The model under review builds one solid part; all positions refer to its coordinate system, in mm. Coordinates: 2 decimals unless noted, no trailing zeros. Write each loop counter-clockwise with the first axis right and the second up, starting at its lowest first coordinate (ties: lowest second). Pieces come first, ordered by that corner, then holes. Notation, with made-up numbers: (50, -3) - (67, -3) arc R33 ccw to (67, 36) - close; hole circle Ø3 at (49.5, 25.25). An arc over 180 degrees is marked (long way). Return JSON: item names as keys, results as strings. Group by question number.
(1) To check wall thickness, follow L1, parallel to X at y = -130, z = 2.35; L2, parallel to Y at x = -28.25, z = 1.2; L3, parallel to Y at x = -85.25, z = 0.8. State the ranges of each line that lie inside material, in increasing order. Write a range as from..to.
(2) We need section A-A on x = 55.5. State the section outline as (y, z) points.
(3) We need section C-C on x = -6. State the section outline as (y, z) points, then the cut area to 3 significant figures.
(4) For pin 1 Ø2.5 at (x, y) = (-85.25, -130) entering from +Z; pin 2 Ø5 at (x, y) = (85.25, 0) entering from +Z, all flat-tipped, find the tip position at first contact; note any pin that passes through.
(5) We need section B-B on z = 0.6. Give the number of separate pieces and of enclosed holes in the cut face, then the cut area to 3 significant figures.
(6) Draft analysis for pull direction Y (two halves, no side actions). For faces 1 (the face through (-1, 2, 3)), 2 (the face through (-1.951, -81.214, 1.479)), state which applies: released by +Y, released by -Y, zero draft, split by the parting line, or undercut.
```python
from build123d import *

# Parameters (mm, degrees)
F1_W      = 190.5
F1_H      = 320
F2_DEPTH  = 3
F4_D      = 4.2
F4_DEPTH  = 4
F4_TIP    = 1.2618073
F6_D      = 3.2
F6_DEPTH  = 4
F6_TIP    = 0.9613769904
F7_W      = 150.5
F7_H      = 20
F8_DEPTH  = 25
F9_R      = 9
F10_DEPTH = 3


# Not quite as in the source:
# - a pattern or mirror of a feature is missing from the dataset's text; its kind, count and spacing are read off the source's solid


with BuildPart() as f2:
    # F1 (on Top) → F2 (new body)
    with BuildSketch(Plane.XY):
        Rectangle(F1_W, F1_H)
    extrude(amount=F2_DEPTH)

    # F4
    with Locations(Plane.XY.offset(3)):
        with Locations((-85.25, 130), (-85.25, 0), (-85.25, -130)):
            f4 = Hole(F4_D / 2, depth=F4_DEPTH)
            with Locations((0, 0, -(F4_DEPTH + F4_TIP / 2))):  # 118° drill point
                Cone(0, F4_D / 2, F4_TIP, mode=Mode.SUBTRACT)

    # F4_copies: F4 across plane
    add(f4.mirror(Plane(origin=(0, 0, 0), x_dir=(0, 0, 1), z_dir=(1, 0, 0))), mode=Mode.SUBTRACT)

    # F6
    with Locations(Plane.XY.offset(3)):
        with Locations((-58.25, 87.5), (-58.25, 59.5), (-28.25, 59.5), (-28.25, 87.5)):
            Hole(F6_D / 2, depth=F6_DEPTH)
            with Locations((0, 0, -(F6_DEPTH + F6_TIP / 2))):  # 118° drill point
                Cone(0, F6_D / 2, F6_TIP, mode=Mode.SUBTRACT)

    # F7 (on face) → F8 (cut)
    with BuildSketch(Plane.XY.offset(3)):
        with Locations((0, -125)):
            Rectangle(F7_W, F7_H)
    extrude(amount=-F8_DEPTH, mode=Mode.SUBTRACT)

    # F9 (on face) → F10 (cut, through all)
    with BuildSketch(Plane(origin=(0, 0, 0), x_dir=(1, 0, 0), z_dir=(0, 0, -1))):
        with Locations((0, 90)):
            Circle(F9_R)
    extrude(amount=-F10_DEPTH, mode=Mode.SUBTRACT)


solid = f2.part
```
Ans:
{
 "1": {"L1": "-95.25..-87.35, -83.15..-75.25, 75.25..83.15, 87.35..95.25", "L2": "-160..-135, -115..57.9, 61.1..85.9, 89.1..160", "L3": "-160..-132.1, -127.9..-2.1, 2.1..127.9, 132.1..160"},
 "2": {"outline": "(-160, 0) - (-135, 0) - (-135, 3) - (-160, 3) - close; (-115, 0) - (160, 0) - (160, 3) - (-115, 3) - close"},
 "3": {"outline": "(-160, 0) - (-135, 0) - (-135, 3) - (-160, 3) - close; (-115, 0) - (-96.71, 0) - (-96.71, 3) - (-115, 3) - close; (-83.29, 0) - (160, 0) - (160, 3) - (-83.29, 3) - close", "area": "860 mm²"},
 "4": {"pin 1": "through", "pin 2": "z = 3"},
 "5": {"separate pieces": "1", "enclosed holes": "12", "area": "57,600 mm²"},
 "6": {"face 1": "zero draft", "face 2": "undercut"}
}
